Autodesk Fusion 360 part; units mm, degrees
sketch "Sketch1" plane through (0, 0, 0) normal (0, 1, 0) x (1, 0, 0)
  circle A0 centre (0, 0) radius 17.5
  circle A1 centre (0, 0) radius 14
  dimension "d1" = 35
  dimension "d2" = 28
extrude "Extrude1" add sketch "Sketch1" along normal blind 10
sketch "Sketch2" plane through (0, 10, 0) normal (0, 1, 0) x (-1, 0, 0)
  circle A0 centre (0, 0) radius 14
  circle A1 centre (0, 0) radius 17.5
  line L0 (-14, -0.0032) -> (-17.5, -0.0032)
  circle A2 centre (-15.75, -0.0032) radius 0.75
  dimension "d5" = 3.5
  dimension "d6" = 1.5
extrude "Extrude2" cut sketch "Sketch2" against normal blind 10 contours L0 A2 | L0 A2
pattern_circular "C-Pattern1" count 16 over 360 about axis through (0, 1.75, 0) along (0, 1, 0) of "Extrude2"
Input: part model. Units: mm. Frame: model coordinates. Coordinates: 2 decimals unless noted, no trailing zeros. Loops run counter-clockwise (first coordinate to the right, second up) from the corner with the lowest first, then second, coordinate; pieces in that order, holes last. Notation, with made-up numbers: (85.25, 23.25) -> (139.25, 23.25) arc R13 cw to (139.25, 42.25) -> close; hole circle Ø7 at (-35.75, 50). An arc over 180 degrees is marked (long way). Use a Markdown table: item, result.
1) Pull-direction query (Z, two-part tool) for faces 1 (the cylindrical face through (-13.887, 4.93, -10.648)), 2 (the cylindrical face through (-5.959, 5.07, 13.805)), 3 (the flat face through (-12, 10, -8)); classes: released by +Z, released by -Z, zero draft, split by the parting line, or undercut.
Results found:
| item | result |
|---|---|
| face 1 | split by the parting line |
| face 2 | undercut |
| face 3 | zero draft |
2) Cut plane B-B (z = -13). Return the cut outline in (x, y), then the cut area to 3 significant figures.
Results found:
| item | result |
|---|---|
| outline | (-11.72, 0) -> (-5.2, 0) -> (-5.2, 10) -> (-11.72, 10) -> close; (5.2, 0) -> (11.72, 0) -> (11.72, 10) -> (5.2, 10) -> close |
| area | 130 mm2 |
3) Material intervals for line 1 along Z through (x, y) = (-11, 6.5); line 2 along X through (y, z) = (9.5, -0.5); line 3 along Z through (x, y) = (-2, 9), sorted ascending. Write a range as from..to.
Results found:
| item | result |
|---|---|
| line 1 | z = -13.61..-11.87, -10.4..-8.66, 8.66..10.4, 11.88..13.61 |
| line 2 | x = -17.49..-16.31, -15.19..-13.99, 13.99..15.19, 16.31..17.49 |
| line 3 | z = -17.39..-13.86, 13.86..17.39 |
4) Contact query for flat-ended pins moving along their axis: pin 1 (0.9 mm diameter, centred on x = 14.55, z = 6.02, fed in from -Y); pin 2 (5 mm diameter, centred on x = 9.5, y = 6, fed in from -Z). Output: stop coordinate, or through.
Results found:
| item | result |
|---|---|
| pin 1 | passes through |
| pin 2 | stops at z = -16.04 |
5) Cut plane A-A (x = 15.75). Return the cut outline in (y, z).
Results found:
| item | result |
|---|---|
| outline | (0, -7.63) -> (10, -7.63) -> (10, -0.75) -> (0, -0.75) -> close; (0, 0.75) -> (10, 0.75) -> (10, 7.63) -> (0, 7.63) -> close |
